The listing builds one solid part. Answer for the finished solid, in the listing's coordinates (mm). Face numbers are marked on the shaded views. Give positions to 0.01 mm unless a question says otherwise; leave off trailing zeros. Write each loop counter-clockwise with the first axis right and the second up, starting at its lowest first coordinate (ties: lowest second). Pieces come first, ordered by that corner, then holes. Notation, with made-up numbers: (1.5, 18) - (38.5, 18) arc R9 cw to (38.5, 27) - close; hole circle Ø2 at (-9, 40). An arc over 180 degrees is marked (long way). Answer in a Markdown table with one row per item. Add a question column.
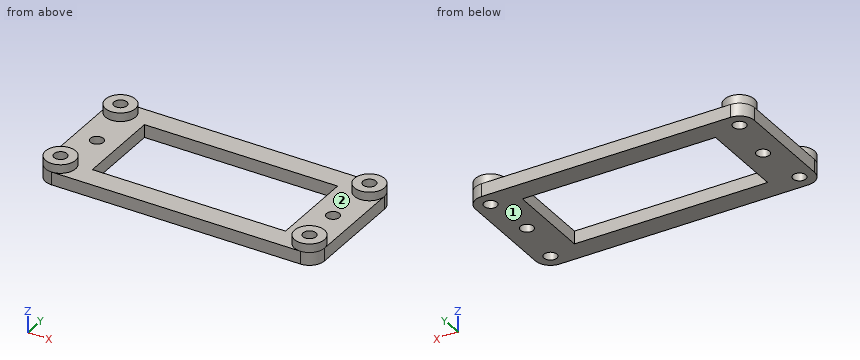
Autodesk Fusion 360 part; units mm, degrees
sketch "Sketch1" plane through (0, 0, 0) normal (0, 0, 1) x (1, 0, 0)
  line L0 (-32.5, 15) -> (32.5, 15)
  line L1 (32.5, 15) -> (32.5, -15)
  line L2 (32.5, -15) -> (-32.5, -15)
  line L3 (-32.5, -15) -> (-32.5, 15)
  line L4 (-32.5, 15) -> (32.5, -15) construction
  line L5 (32.5, 15) -> (-32.5, -15) construction
  circle A0 centre (-29, 11.5) radius 1.5
  circle A1 centre (29, 11.5) radius 1.5
  circle A2 centre (-29, -11.5) radius 1.5
  circle A3 centre (29, -11.5) radius 1.5
  dimension "d1" = 65
  dimension "d2" = 30
  dimension "d3" = 3
  dimension "d4" = 3.5
  dimension "d5" = 3.5
  dimension "d8" = 58
  dimension "d9" = -23
extrude "Extrude1" add sketch "Sketch1" along normal blind 3
sketch "Sketch2" plane through (0, 0, 3) normal (0, 0, 1) x (-1, 0, 0)
  circle A0 centre (-29, -11.5) radius 1.5
  circle A1 centre (29, 11.5) radius 1.5
  circle A2 centre (29, -11.5) radius 1.5
  circle A3 centre (-29, 11.5) radius 1.5
  line L0 (32.5, 15) -> (-32.5, 15)
  line L1 (-32.5, 15) -> (-32.5, -15)
  line L2 (-32.5, -15) -> (32.5, -15)
  line L3 (32.5, -15) -> (32.5, 15)
  circle A4 centre (29, -11.5) radius 3.5
  circle A5 centre (-29, -11.5) radius 3.5
  circle A6 centre (29, 11.5) radius 3.5
  circle A7 centre (-29, 11.5) radius 3.5
  dimension "d14" = -58
  dimension "d15" = 23
extrude "Extrude2" add sketch "Sketch2" along normal blind 2 contours A6 | A7 | A4 | A5
fillet "Fillet1" radius 3.5 4 edges at (-32.5, -15, 1.5) (-32.5, 15, 1.5) (32.5, -15, 1.5) (32.5, 15, 1.5)
sketch "Sketch3" plane through (0, 0, 3) normal (0, 0, 1) x (-1, 0, 0)
  arc A0 (-29, -15) -> (-32.5, -11.5) centre (-29, -11.5) ccw
  line L0 (-29, -15) -> (29, -15)
  arc A1 (32.5, -11.5) -> (29, -15) centre (29, -11.5) ccw
  line L1 (32.5, -11.5) -> (32.5, 11.5)
  arc A2 (29, 15) -> (32.5, 11.5) centre (29, 11.5) ccw
  line L2 (29, 15) -> (-29, 15)
  arc A3 (-32.5, 11.5) -> (-29, 15) centre (-29, 11.5) ccw
  line L3 (-32.5, 11.5) -> (-32.5, -11.5)
  line L4 (25.5013, -11.5936) -> (-25.5013, 11.5936) construction
  line L5 (-25.5013, -11.5936) -> (25.5013, 11.5936) construction
  circle A4 centre (27.5, 0) radius 1.5
  circle A5 centre (-27.5, 0) radius 1.5
  line L6 (22.5, -10) -> (-22.5, -10)
  line L7 (-22.5, -10) -> (-22.5, 10)
  line L8 (-22.5, 10) -> (22.5, 10)
  line L9 (22.5, 10) -> (22.5, -10)
  line L10 (22.5, -10) -> (-22.5, 10) construction
  line L11 (-22.5, -10) -> (22.5, 10) construction
  dimension "d20" = 3
  dimension "d21" = 3
  dimension "d22" = 27.5
  dimension "d23" = 27.5
  dimension "d24" = 5
  dimension "d25" = 5
  dimension "d26" = 5
extrude "Extrude3" cut sketch "Sketch3" against normal up to surface (3 mm away) contours A4 | A5 | L6 L7 L8 L9
equation "d24 = d25"
equation "d26 = d25"
1. Given pin 1 Ø10 at (x, y) = (-12.5, -6.5) entering from +Z; pin 2 Ø2.5 at (x, y) = (-27.5, 0) entering from -Z, each flat-ended and moving along its own axis, determine where each tip first touches the part or whether it passes through.
2. Section D-D (y = -4) is taken. Give the vertices of the cut face in (x, z), and give its area (3 significant figures).
3. Section B-B (y = 0) is taken. Give the vertices of the cut face in (x, z), and give its area (3 significant figures).
4. Section C-C (z = 1.2) is taken. Give the vertices of the cut face in (x, y), and give its area (3 significant figures).
5. Straight lines are drawn through the part: L1, parallel to X at y = 0, z = 2.05; L2, parallel to Y at x = -29, z = 3.8; L3, parallel to X at y = -11.5, z = 3.4. For each, find the intervals that lie inside material, in ascending order. Write a range as [from, to].
6. Section A-A (x = -15) is taken. Give the vertices of the cut face in (y, z).
7. The mould has two halves that part along Y. Classify the marked faces 1 and 2: +Y half, -Y half, draft (parallel to the pull), parting line (faces both ways), or undercut.
Geometry check:
| question | item | result |
|---|---|---|
| 1 | pin 1 | z = 3 |
| 1 | pin 2 | through |
| 2 | outline | (-32.5, 0) - (-22.5, 0) - (-22.5, 3) - (-32.5, 3) - close; (22.5, 0) - (32.5, 0) - (32.5, 3) - (22.5, 3) - close |
| 2 | area | 60.0 mm² |
| 3 | outline | (-32.5, 0) - (-29, 0) - (-29, 3) - (-32.5, 3) - close; (-26, 0) - (-22.5, 0) - (-22.5, 3) - (-26, 3) - close; (22.5, 0) - (26, 0) - (26, 3) - (22.5, 3) - close; (29, 0) - (32.5, 0) - (32.5, 3) - (29, 3) - close |
| 3 | area | 42.0 mm² |
| 4 | outline | (-32.5, -11.5) arc R3.5 ccw to (-29, -15) - (29, -15) arc R3.5 ccw to (32.5, -11.5) - (32.5, 11.5) arc R3.5 ccw to (29, 15) - (-29, 15) arc R3.5 ccw to (-32.5, 11.5) - close; hole circle Ø3 at (-29, -11.5); hole circle Ø3 at (-29, 11.5); hole circle Ø3 at (-27.5, 0); hole (-22.5, -10) - (22.5, -10) - (22.5, 10) - (-22.5, 10) - close; hole circle Ø3 at (27.5, 0); hole circle Ø3 at (29, -11.5); hole circle Ø3 at (29, 11.5) |
| 4 | area | 997 mm² |
| 5 | L1 | [-32.5, -29], [-26, -22.5], [22.5, 26], [29, 32.5] |
| 5 | L2 | [-15, -13], [-10, -8], [8, 10], [13, 15] |
| 5 | L3 | [-32.5, -30.5], [-27.5, -25.5], [25.5, 27.5], [30.5, 32.5] |
| 6 | outline | (-15, 0) - (-10, 0) - (-10, 3) - (-15, 3) - close; (10, 0) - (15, 0) - (15, 3) - (10, 3) - close |
| 7 | face 1 | draft |
| 7 | face 2 | undercut |
